Can you work these out from the model? Positions are in its coordinate system, mm. Face numbers are marked on the shaded views. A direction names the side the tool comes from. Round coordinates to 2 decimals unless told otherwise and drop trailing zeros. Order: outer loops, then holes, each group sorted by start corner. A loop starts at its lowest first (then second) coordinate and runs counter-clockwise, first axis right, second up. Notation, with made-up numbers: (53.5, -0.75) -> (80.5, -0.75) arc R9 ccw to (80.5, 8.25) -> close; hole circle Ø1 at (61, 68.25). An arc over 180 degrees is marked (long way). One line per item, written item: value.
```python
from build123d import *

# Parameters (mm, degrees)
SKETCH_1_R                = 9
EXTRUDE_1_DEPTH           = 4
SKETCH_2_R                = 14
EXTRUDE_2_DEPTH           = 3
SKETCH_3_R                = 6.25
CUT_EXTRUDE_1_DEPTH       = 2.1
HOLE_WIZARD_1_D           = 5.5
HOLE_WIZARD_1_CSINK_D     = 11.2
HOLE_WIZARD_1_CSINK_ANGLE = 90
CHAMFER_1_SIZE            = 0.5


with BuildPart() as part:
    # 草图1 → 凸台-拉伸1 (new body)
    with BuildSketch(Plane.XY):
        Circle(SKETCH_1_R)
    extrude(amount=EXTRUDE_1_DEPTH)

    # 草图2 → 凸台-拉伸2 (add)
    with BuildSketch(Plane(origin=(0, 0, 0), x_dir=(-1, 0, 0), z_dir=(0, 0, -1))):
        Circle(SKETCH_2_R)
    extrude(amount=EXTRUDE_2_DEPTH)

    # 草图3 → 切除-拉伸1 (cut)
    with BuildSketch(Plane.XY.offset(4)):
        Circle(SKETCH_3_R)
    extrude(amount=-CUT_EXTRUDE_1_DEPTH, mode=Mode.SUBTRACT)

    # 打孔尺寸根据开槽半沉头木螺钉的类型1 (through all)
    with Locations(Plane(origin=(0, 0, -3), x_dir=(-1, 0, 0), z_dir=(0, 0, -1))):
        with Locations((0, 0)):
            CounterSinkHole(HOLE_WIZARD_1_D / 2, HOLE_WIZARD_1_CSINK_D / 2, counter_sink_angle=HOLE_WIZARD_1_CSINK_ANGLE)

    # 倒角1
    chamfer_1_edges = [part.edges().sort_by_distance(p)[0] for p in [
        (-9, 0, 4),
        (14, 0, 0),
        (14, 0, -3),
    ]]
    chamfer(chamfer_1_edges, length=CHAMFER_1_SIZE)


solid = part.part
```
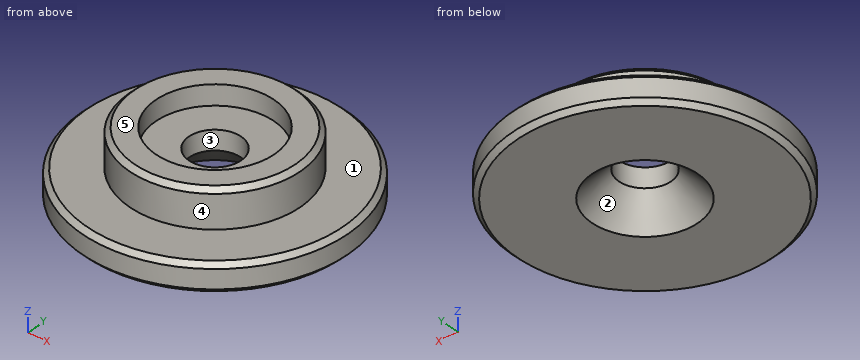
Q1. I want a section at D-D on z = 1. List the corners of the cut face in (x, y) for me.
Answers below:
outline: circle Ø18 at (0, 0); hole circle Ø5.5 at (0, 0)
Q2. I want a section at C-C on z = -1. List the corners of the cut face in (x, y) for me, plus the area to 3 significant figures.
Answers below:
outline: circle Ø28 at (0, 0); hole circle Ø7.2 at (0, 0)
area: 575 mm^2
Q3. I want a section at A-A on y = 0. List the corners of the cut face in (x, z) for me.
Answers below:
outline: (-14, -2.5) -> (-13.5, -3) -> (-5.6, -3) -> (-2.75, -0.15) -> (-2.75, 1.9) -> (-6.25, 1.9) -> (-6.25, 4) -> (-8.5, 4) -> (-9, 3.5) -> (-9, 0) -> (-13.5, 0) -> (-14, -0.5) -> close; (2.75, -0.15) -> (5.6, -3) -> (13.5, -3) -> (14, -2.5) -> (14, -0.5) -> (13.5, 0) -> (9, 0) -> (9, 3.5) -> (8.5, 4) -> (6.25, 4) -> (6.25, 1.9) -> (2.75, 1.9) -> close
Q4. We'd pull the mould along X, two halves only. Please class the marked faces 3, 4 and 5: released by +X, released by -X, zero draft, split by the parting line, or undercut.
Answers below:
face 3: undercut
face 4: split by the parting line
face 5: zero draft
Q5. On a 3-axis mill with a long thin cutter (end or side, diameter ignored), from which of +Z, -Z, +X, -X, +Y, -Y can I reach the whole of each face in a straight line? I mean the marked faces 1 and 2. Say none if no direction works.
Answers below:
face 1: +Z
face 2: -Z
Q6. Please list where these lines run through material, in increasing order: line 1 along Y through (x, z) = (0, 0.75); line 2 along Z through (x, y) = (9.75, 1.5); line 3 along X through (y, z) = (5, 3).
Answers below:
line 1: -9 to -2.75, 2.75 to 9
line 2: -3 to 0
line 3: -7.48 to -3.75, 3.75 to 7.48
Q7. Will these pins go through, and if not, where does the flat tip stop? pin 1 Ø10 at (x, y) = (0, 0) entering from -Z; pin 2 Ø4 at (x, z) = (-10.5, -0.5) entering from -Y.
Answers below:
pin 1: z = -2.4
pin 2: y = -11.12
